The listing builds one solid part. Answer for the finished solid, in the listing's coordinates (mm). A direction names the side the tool comes from. Give positions to 0.01 mm unless a question says otherwise; leave off trailing zeros. Order: outer loops, then holes, each group sorted by start corner. A loop starts at its lowest first (then second) coordinate and runs counter-clockwise, first axis right, second up. Notation, with made-up numbers: (34.25, 36.25) - (67.25, 36.25) arc R10 cw to (67.25, 53.25) - close; hole circle Ø5 at (-26.5, -7). An arc over 180 degrees is marked (long way). Answer as a JSON object with one key per item and string values. Group by question number.
Q1. A cutting plane is placed at D-D, the plane y = -12. Give the vertices of the cut face in (x, z), and give its area (3 significant figures).
Q2. The mould has two halves that part along X. Classify faces 4 (the face through (17.57, 17.66, -0.21)), 5 (the face through (-17, 15.57, 21.47)), 6 (the face through (0, 0, 43.7)), 7 (the face through (15, -15, 19.5)): released by +X, released by -X, zero draft, split by the parting line, or undercut.
Q3. For faces 1 (the face through (-17, -15.43, 21.47)), 2 (the face through (-17.66, 17.57, -0.21)), 3 (the face through (-17.57, -17.66, -0.21)), determine the directions among +Z, -Z, +X, -X, +Y, -Y from which every point of the face is accessible in a straight line to the end or side of a thin tool.
Q4. A cutting plane is placed at A-A, the plane y = 0. Give the vertices of the cut face in (x, z), and give its area (3 significant figures).
Q5. A cutting plane is placed at C-C, the plane x = 4. Give the vertices of the cut face in (y, z), and give its area (3 significant figures).
Q6. Given pin 1 (3.5 mm diameter, centred on x = 15, y = -15.5, fed in from -Z); pin 2 (5 mm diameter, centred on x = 15.5, y = 15.5, fed in from +Z); pin 3 (1.5 mm diameter, centred on x = -16, y = 16, fed in from +Z); pin 4 (12.5 mm diameter, centred on x = -3.5, y = -9.5, fed in from +Z), each flat-ended and moving along its own axis, determine where each tip first touches the part or whether it passes through.
Q7. Consider line 1 (Y direction, x = -15.5, z = -21.7); line 2 (Y direction, x = -16, z = 22); line 3 (Z direction, x = -9, y = -7). Determine where each line is inside the solid, lowest interval first.
Q8. A cutting plane is placed at B-B, the plane z = 5. Give the vertices of the cut face in (x, y).
from build123d import *

# Parameters (mm, degrees)
BOSS_EXTRUDE1_DEPTH      = 23.5
BOSS_EXTRUDE1_DEPTH_BACK = 23.5
SKETCH1_R                = 11
SKETCH1_R_2              = 1.5
CUT_EXTRUDE1_DEPTH       = 15
CUT_EXTRUDE1_DEPTH_BACK  = 15
BOSS_EXTRUDE2_DEPTH      = 25.5
BOSS_EXTRUDE2_DEPTH_BACK = 23.5
SKETCH1_9_R              = 11
SKETCH1_9_R_2            = 2.5
BOSS_EXTRUDE3_DEPTH      = 43.7
BOSS_EXTRUDE3_DEPTH_BACK = 23
SKETCH1_10_R             = 2.5
BOSS_EXTRUDE4_DEPTH      = 19.5
BOSS_EXTRUDE4_DEPTH_BACK = 19.5
SKETCH1_11_R             = 1.5


with BuildPart() as part:
    # Sketch1 → Boss-Extrude1 (new, two sides: drawn at the far end of the back side and taken through both)
    with BuildSketch(Plane.XY.offset(-BOSS_EXTRUDE1_DEPTH_BACK)):
        Polygon((-16.907359313, 21.15), (-21.15, 16.907359313), (-21.15, -16.907359313), (-16.907359313, -21.15), (16.907359313, -21.15), (21.15, -16.907359313), (21.15, 16.907359313), (16.907359313, 21.15), align=None)
        Circle(SKETCH1_R, mode=Mode.SUBTRACT)
        with Locations((15.5, 15.5)):
            Circle(SKETCH1_R_2, mode=Mode.SUBTRACT)
        with Locations((-15.5, 15.5)):
            Circle(SKETCH1_R_2, mode=Mode.SUBTRACT)
        with Locations((-15.5, -15.5)):
            Circle(SKETCH1_R_2, mode=Mode.SUBTRACT)
        with Locations((15.5, -15.5)):
            Circle(SKETCH1_R_2, mode=Mode.SUBTRACT)
    extrude(amount=BOSS_EXTRUDE1_DEPTH + BOSS_EXTRUDE1_DEPTH_BACK)

    # Sketch1<8> → Cut-Extrude1 (cut, two sides: drawn at the far end of the back side and taken through both)
    with BuildSketch(Plane.XY.offset(-CUT_EXTRUDE1_DEPTH_BACK)):
        Polygon((-21, 14.228932188), (-21.15, 14.078932188), (-21.15, -14.078932188), (-21, -14.228932188), align=None)
        Polygon((-14.228932188, 21), (-17.057359313, 21), (-21, 17.057359313), (-21, 14.228932188), align=None)
        Polygon((14.078932188, 21.15), (-14.078932188, 21.15), (-14.228932188, 21), (14.228932188, 21), align=None)
        Polygon((17.057359313, 21), (14.228932188, 21), (21, 14.228932188), (21, 17.057359313), align=None)
        Polygon((21.15, 14.078932188), (21, 14.228932188), (21, -14.228932188), (21.15, -14.078932188), align=None)
        Polygon((21, -17.057359313), (21, -14.228932188), (14.228932188, -21), (17.057359313, -21), align=None)
        Polygon((14.228932188, -21), (-14.228932188, -21), (-14.078932188, -21.15), (14.078932188, -21.15), align=None)
        Polygon((17.057359313, -21), (14.228932188, -21), (14.078932188, -21.15), (16.907359313, -21.15), align=None)
        Polygon((21.15, -14.078932188), (21, -14.228932188), (21, -17.057359313), (21.15, -16.907359313), align=None)
        Polygon((16.907359313, 21.15), (14.078932188, 21.15), (14.228932188, 21), (17.057359313, 21), align=None)
        Polygon((21, 17.057359313), (21, 14.228932188), (21.15, 14.078932188), (21.15, 16.907359313), align=None)
        Polygon((-14.078932188, 21.15), (-16.907359313, 21.15), (-17.057359313, 21), (-14.228932188, 21), align=None)
        Polygon((-21, 17.057359313), (-21.15, 16.907359313), (-21.15, 14.078932188), (-21, 14.228932188), align=None)
        Polygon((-14.228932188, -21), (-21, -14.228932188), (-21, -17.057359313), (-17.057359313, -21), align=None)
        Polygon((-21, -14.228932188), (-21.15, -14.078932188), (-21.15, -16.907359313), (-21, -17.057359313), align=None)
        Polygon((-14.078932188, -21.15), (-14.228932188, -21), (-17.057359313, -21), (-16.907359313, -21.15), align=None)
    extrude(amount=CUT_EXTRUDE1_DEPTH + CUT_EXTRUDE1_DEPTH_BACK, mode=Mode.SUBTRACT)

    # Sketch1<9> → Boss-Extrude2 (add, two sides: drawn at the far end of the back side and taken through both)
    with BuildSketch(Plane.XY.offset(-BOSS_EXTRUDE2_DEPTH_BACK)):
        Circle(SKETCH1_9_R)
        Circle(SKETCH1_9_R_2, mode=Mode.SUBTRACT)
    extrude(amount=BOSS_EXTRUDE2_DEPTH + BOSS_EXTRUDE2_DEPTH_BACK)

    # Sketch1<10> → Boss-Extrude3 (add, two sides: drawn at the far end of the back side and taken through both)
    with BuildSketch(Plane.XY.offset(-BOSS_EXTRUDE3_DEPTH_BACK)):
        Circle(SKETCH1_10_R)
    extrude(amount=BOSS_EXTRUDE3_DEPTH + BOSS_EXTRUDE3_DEPTH_BACK)

    # Sketch1<11> → Boss-Extrude4 (add, two sides: drawn at the far end of the back side and taken through both)
    with BuildSketch(Plane.XY.offset(-BOSS_EXTRUDE4_DEPTH_BACK)):
        with Locations((-15.5, -15.5)):
            Circle(SKETCH1_11_R)
        with Locations((-15.5, 15.5)):
            Circle(SKETCH1_11_R)
        with Locations((15.5, 15.5)):
            Circle(SKETCH1_11_R)
        with Locations((15.5, -15.5)):
            Circle(SKETCH1_11_R)
    extrude(amount=BOSS_EXTRUDE4_DEPTH + BOSS_EXTRUDE4_DEPTH_BACK)


solid = part.part
Reply:
{
 "1": {"outline": "(-21.15, -23.5) - (21.15, -23.5) - (21.15, -15) - (21, -15) - (21, 15) - (21.15, 15) - (21.15, 23.5) - (-21.15, 23.5) - (-21.15, 15) - (-21, 15) - (-21, -15) - (-21.15, -15) - close", "area": "1,980 mm^2"},
 "2": {"face 4": "released by +X", "face 5": "undercut", "face 6": "zero draft", "face 7": "undercut"},
 "3": {"face 1": "+Z", "face 2": "-X, +Y", "face 3": "-X, -Y"},
 "4": {"outline": "(-21.15, -23.5) - (-2.5, -23.5) - (-2.5, -23) - (2.5, -23) - (2.5, -23.5) - (21.15, -23.5) - (21.15, -15) - (21, -15) - (21, 15) - (21.15, 15) - (21.15, 23.5) - (11, 23.5) - (11, 25.5) - (2.5, 25.5) - (2.5, 43.7) - (-2.5, 43.7) - (-2.5, 25.5) - (-11, 25.5) - (-11, 23.5) - (-21.15, 23.5) - (-21.15, 15) - (-21, 15) - (-21, -15) - (-21.15, -15) - close", "area": "2,110 mm^2"},
 "5": {"outline": "(-21.15, -23.5) - (21.15, -23.5) - (21.15, -15) - (21, -15) - (21, 15) - (21.15, 15) - (21.15, 23.5) - (10.25, 23.5) - (10.25, 25.5) - (-10.25, 25.5) - (-10.25, 23.5) - (-21.15, 23.5) - (-21.15, 15) - (-21, 15) - (-21, -15) - (-21.15, -15) - close", "area": "2,020 mm^2"},
 "6": {"pin 1": "stops at z = -23.5", "pin 2": "stops at z = 23.5", "pin 3": "stops at z = 19.5", "pin 4": "stops at z = 25.5"},
 "7": {"line 1": "y = -21.15 to -17, -14 to 14, 17 to 21.15", "line 2": "y = -21.15 to -16.91, -14.09 to 14.09, 16.91 to 21.15", "line 3": "z = -23.5 to 23.5"},
 "8": {"outline": "(-21, -14.23) - (-14.23, -21) - (14.23, -21) - (21, -14.23) - (21, 14.23) - (14.23, 21) - (-14.23, 21) - (-21, 14.23) - close"}
}
